```python
from build123d import *

# Parameters (mm, degrees)
BOSS_EXTRUDE1_DEPTH   = 9.525
BOSS_EXTRUDE2_DEPTH   = 5.969
CAVITY1_START         = -5.969
CAVITY1_OUTLINE_R     = 4.445
CAVITY1_OUTLINE_R_2   = 1.143
CAVITY1_DEPTH         = 10.16
CAVITY1_START_2       = 4.191
CAVITY1_2_OUTLINE_R   = 7.239
CAVITY1_2_OUTLINE_R_2 = 1.143
CAVITY1_2_DEPTH       = 5.334
CAVITY1_3_OUTLINE_R   = 4.445
CAVITY1_3_DEPTH       = 3.048
CAVITY1_4_OUTLINE_R   = 6.35
CAVITY1_4_OUTLINE_R_2 = 4.445
CAVITY1_4_DEPTH       = 1.778
CAVITY1_START_3       = 6.223
CAVITY1_5_OUTLINE_R   = 1.905
CAVITY1_5_OUTLINE_R_2 = 1.143
CAVITY1_5_DEPTH       = 3.302
CAVITY1_6_OUTLINE_R   = 2.286
CAVITY1_6_DEPTH       = 1.27
CAVITY1_START_4       = 7.239
CAVITY1_7_DEPTH       = 0.254


# Read off the part's stored shape, not the designer's step: Cavity1
with BuildPart() as part:
    # Sketch1 → Boss-Extrude1 (new body)
    with BuildSketch(Plane.XY):
        Polygon((-41.443198843, -69.435406513), (-16.043198843, -69.435406513), (-16.043198843, -83.405406513), (-6.518198843, -83.405406513), (-6.518198843, -52.448144489), (33.310925875, 30.495820593), (2.972453908, 45.064147324), (-30.788372585, -25.242615218), (-22.202012594, -29.365726557), align=None)
    extrude(amount=BOSS_EXTRUDE1_DEPTH)

    # Sketch2 → Boss-Extrude2 (add)
    with BuildSketch(Plane(origin=(0, 0, 0), x_dir=(-1, 0, 0), z_dir=(0, 0, -1))):
        Polygon((-2.972453908, 45.064147324), (-33.310925875, 30.495820593), (-8.022509662, -22.167187349), (22.315962304, -7.598860618), align=None)
    extrude(amount=BOSS_EXTRUDE2_DEPTH)

    # Cavity1 outline → Cavity1 (cut)
    with BuildSketch(Plane.XY.offset(CAVITY1_START)):
        with BuildLine():
            ThreePointArc((11.508743469, 8.573215544), (6.212154418, 12.936782386), (-0.504959238, 14.342113414))
            ThreePointArc((-0.504959238, 14.342113414), (-3.150914892, 17.086873862), (-4.643828287, 13.578882864))
            ThreePointArc((-4.643828287, 13.578882864), (-12.936782386, 6.212154417), (-13.500892619, -4.86591199))
            ThreePointArc((-13.500892619, -4.86591199), (-15.305202325, -8.224372608), (-11.508743469, -8.573215544))
            ThreePointArc((-11.508743469, -8.573215544), (-6.212154418, -12.936782386), (0.504959238, -14.342113414))
            ThreePointArc((0.504959238, -14.342113414), (3.150914892, -17.086873862), (4.643828287, -13.578882864))
            ThreePointArc((4.643828287, -13.578882864), (12.936782386, -6.212154417), (13.500892619, 4.86591199))
            ThreePointArc((13.500892619, 4.86591199), (15.305202325, 8.224372608), (11.508743469, 8.573215544))
        make_face()
        with Locations((10.994963571, 22.896959975)):
            Circle(CAVITY1_OUTLINE_R)
        with Locations((2.35982247, 37.187095529)):
            Circle(CAVITY1_OUTLINE_R_2)
        with Locations((27.546478442, 25.092635602)):
            Circle(CAVITY1_OUTLINE_R_2)
        with Locations((8.635141101, -14.290135555)):
            Circle(CAVITY1_OUTLINE_R_2)
        with Locations((-16.551514871, -2.195675627)):
            Circle(CAVITY1_OUTLINE_R_2)
    extrude(amount=CAVITY1_DEPTH, mode=Mode.SUBTRACT)

    # Cavity1 2 outline → Cavity1 2 (cut)
    with BuildSketch(Plane.XY.offset(CAVITY1_START_2)):
        Circle(CAVITY1_2_OUTLINE_R)
        with Locations((2.35982247, 37.187095529)):
            Circle(CAVITY1_2_OUTLINE_R_2)
        with Locations((27.546478442, 25.092635602)):
            Circle(CAVITY1_2_OUTLINE_R_2)
        with Locations((8.635141101, -14.290135555)):
            Circle(CAVITY1_2_OUTLINE_R_2)
        with Locations((-16.551514871, -2.195675627)):
            Circle(CAVITY1_2_OUTLINE_R_2)
    extrude(amount=CAVITY1_2_DEPTH, mode=Mode.SUBTRACT)

    # Cavity1 3 outline → Cavity1 3 (cut)
    with BuildSketch(Plane.XY.offset(CAVITY1_START_2)):
        with BuildLine():
            ThreePointArc((2.747559241, 14.085528716), (3.84823725, 8.013935991), (9.274883676, 10.951152168))
            ThreePointArc((9.274883676, 10.951152168), (6.212154418, 12.936782386), (2.747559241, 14.085528716))
        make_face()
        with Locations((10.994963571, 22.896959975)):
            Circle(CAVITY1_3_OUTLINE_R)
    extrude(amount=CAVITY1_3_DEPTH, mode=Mode.SUBTRACT)

    # Cavity1 4 outline → Cavity1 4 (cut)
    with BuildSketch(Plane.XY.offset(CAVITY1_START)):
        with Locations((11.819585838, 24.614231973)):
            Circle(CAVITY1_4_OUTLINE_R)
        with Locations((10.994963571, 22.896959975)):
            Circle(CAVITY1_4_OUTLINE_R_2, mode=Mode.SUBTRACT)
    extrude(amount=CAVITY1_4_DEPTH, mode=Mode.SUBTRACT)

    # Cavity1 5 outline → Cavity1 5 (cut)
    # profile 1 of 4: a face of its own
    with BuildSketch(Plane.XY.offset(CAVITY1_START_3)):
        with Locations((2.35982247, 37.187095529)):
            Circle(CAVITY1_5_OUTLINE_R)
        with Locations((2.35982247, 37.187095529)):
            Circle(CAVITY1_5_OUTLINE_R_2, mode=Mode.SUBTRACT)
    # profile 2 of 4: a face of its own
    with BuildSketch(Plane.XY.offset(CAVITY1_START_3)):
        with Locations((27.546478442, 25.092635602)):
            Circle(CAVITY1_5_OUTLINE_R)
        with Locations((27.546478442, 25.092635602)):
            Circle(CAVITY1_5_OUTLINE_R_2, mode=Mode.SUBTRACT)
    # profile 3 of 4: a face of its own
    with BuildSketch(Plane.XY.offset(CAVITY1_START_3)):
        with Locations((8.635141101, -14.290135555)):
            Circle(CAVITY1_5_OUTLINE_R)
        with Locations((8.635141101, -14.290135555)):
            Circle(CAVITY1_5_OUTLINE_R_2, mode=Mode.SUBTRACT)
    # profile 4 of 4: a face of its own
    with BuildSketch(Plane.XY.offset(CAVITY1_START_3)):
        with Locations((-16.551514871, -2.195675627)):
            Circle(CAVITY1_5_OUTLINE_R)
        with Locations((-16.551514871, -2.195675627)):
            Circle(CAVITY1_5_OUTLINE_R_2, mode=Mode.SUBTRACT)
    extrude(amount=CAVITY1_5_DEPTH, mode=Mode.SUBTRACT)

    # Cavity1 6 outline → Cavity1 6 (cut)
    with BuildSketch(Plane.XY.offset(CAVITY1_START_2)):
        with Locations((13.291518505, 7.142303538)):
            Circle(CAVITY1_6_OUTLINE_R)
        with Locations((-2.736353477, 14.838778038)):
            Circle(CAVITY1_6_OUTLINE_R)
        with Locations((2.736353477, -14.838778038)):
            Circle(CAVITY1_6_OUTLINE_R)
        with Locations((-13.291518505, -7.142303538)):
            Circle(CAVITY1_6_OUTLINE_R)
    extrude(amount=CAVITY1_6_DEPTH, mode=Mode.SUBTRACT)

    # Cavity1 7 outline → Cavity1 7 (cut)
    with BuildSketch(Plane.XY.offset(CAVITY1_START_4)):
        with BuildLine():
            ThreePointArc((2.747559241, 14.085528716), (3.84823725, 8.013935991), (9.274883676, 10.951152168))
            ThreePointArc((9.274883676, 10.951152168), (6.212154418, 12.936782386), (2.747559241, 14.085528716))
        make_face()
    extrude(amount=CAVITY1_7_DEPTH, mode=Mode.SUBTRACT)


solid = part.part
```
Geometry: final body of the model. Coordinates: model frame, mm. A direction names the side the tool comes from. Round coordinates to 2 decimals unless told otherwise and drop trailing zeros. Loops run counter-clockwise (first coordinate to the right, second up) from the corner with the lowest first, then second, coordinate; pieces in that order, holes last.
Item 1: Reachability of faces 1 (the flat face through (-31.69, -49.12, 4.7)), 2 (the flat face through (-29, -69.435, 5)), 3 (the cylindrical face through (12.867, -6.356, -0.96)), 4 (the cylindrical face through (8.486, -13.157, 0.042)) from +Z, -Z, +X, -X, +Y, -Y: full face, straight path, thin tool, end or side. Return the list, or none.
Checked values:
face 1: +Z, -Z, -X
face 2: +Z, -Z, -X, -Y
face 3: -Z
face 4: +Z, -Z
Item 2: Mould query, pull axis X, two halves, no side actions, for faces 5 (the flat face through (5, 11, 7.493)), 6 (the flat face through (-17, -37, 0)), 7 (the flat face through (-6.518, -68, 5)). Classes: released by +X, released by -X, zero draft, split by the parting line, or undercut.
Checked values:
face 5: undercut
face 6: zero draft
face 7: released by +X
Item 3: Section A-A, the plane z = 2. Output: boundary loops of the cut face in (x, y) (3 decimals).
Checked values:
outline: (-41.443, -69.435) - (-16.043, -69.435) - (-16.043, -83.405) - (-6.518, -83.405) - (-6.518, -52.448) - (33.311, 30.496) - (2.972, 45.064) - (-30.788, -25.243) - (-22.202, -29.366) - close; hole circle Ø2.286 at (-16.552, -2.196); hole (-13.501, -4.866) arc R2.286 ccw (long way) to (-11.509, -8.573) arc R14.351 ccw to (0.505, -14.342) arc R2.286 ccw (long way) to (4.644, -13.579) arc R14.351 ccw to (13.501, 4.866) arc R2.286 ccw (long way) to (11.509, 8.573) arc R14.351 ccw to (-0.505, 14.342) arc R2.286 ccw (long way) to (-4.644, 13.579) arc R14.351 ccw to start; hole circle Ø2.286 at (2.36, 37.187); hole circle Ø8.89 at (10.995, 22.897); hole circle Ø2.286 at (8.635, -14.29); hole circle Ø2.286 at (27.546, 25.093)
Item 4: Line query: L1, parallel to Y at x = 2, z = -3; L2, parallel to Y at x = 10.5, z = -2; L3, parallel to X at y = 27, z = -1. Output: solid intervals per line, ascending.
Checked values:
L1: y = -19.28 to -17, 14.21 to 36.1, 38.27 to 43.04
L2: y = -17.01 to -9.78, 9.78 to 18.48, 27.31 to 41.45
L3: x = -5.7 to 9.29, 12.7 to 31.63
Item 5: Contact query for flat-ended pins moving along their axis: P1, Ø2.5, axis at x = 27.55, y = 25.09, coming from the -Z side; P2, Ø4, axis at x = -13.29, y = -7.14, coming from the -Z side; P3, Ø1.5, axis at y = -26.5, z = 4.5, coming from the +X side; P4, Ø3, axis at x = -29, z = 7, coming from the -Y side. Output: stop coordinate, or through.
Checked values:
P1: stops at z = -5.97
P2: stops at z = 5.46
P3: stops at x = 6.3
P4: stops at y = -69.44
Item 6: Section B-B, the plane y = -59. Output: boundary loops of the cut face in (x, z) (3 decimals), plus the area to 3 significant figures.
Checked values:
outline: (-36.432, 0) - (-6.518, 0) - (-6.518, 9.525) - (-36.432, 9.525) - close
area: 285 mm2
